Job drawing, mm, ordinate dimensions from the low corner. One solid piece. A direction names the side the tool comes from. Give positions to 0.01 mm unless a question says otherwise; leave off trailing zeros. Loops run counter-clockwise (first coordinate to the right, second up) from the corner with the lowest first, then second, coordinate; pieces in that order, holes last. Notation, with made-up numbers: M 71.25,15 L 98.25,15 A8 cw 98.25,27 Z; hole C -17.5,73 d9. An arc over 180 degrees is marked long. One line per question, with ' | ' between items.
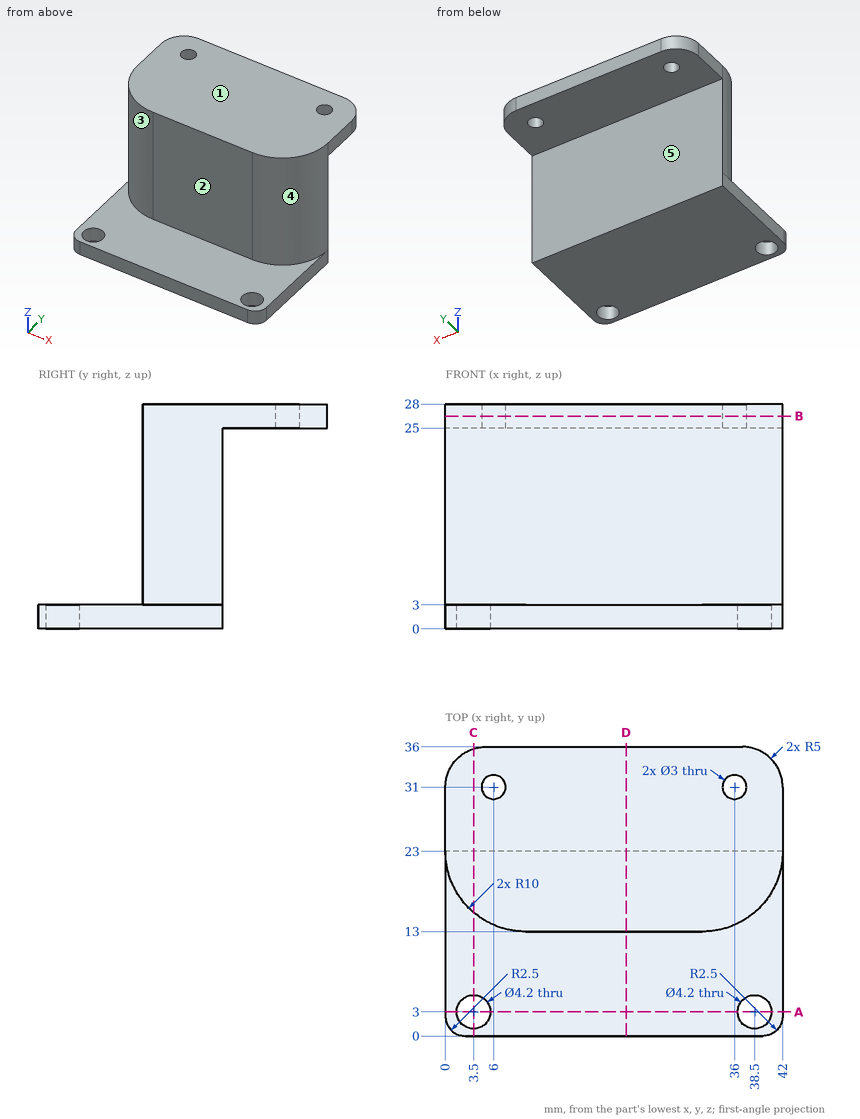
Item 1: Saw through at C-C on x = 3.5. Give the cut face in (y, z), and give its area (3 significant figures).
Conclusion:
outline: M 0,0 L 0.9,0 L 0.9,3 L 0,3 Z; M 5.1,0 L 23,0 L 23,25 L 35.77,25 L 35.77,28 L 15.4,28 L 15.4,3 L 5.1,3 Z | area: 285 mm²
Item 2: Saw through at B-B on z = 26.5. Give the cut face in (x, y), and give its area (3 significant figures).
Conclusion:
outline: M 0,23 A10 ccw 10,13 L 32,13 A10 ccw 42,23 L 42,31 A5 ccw 37,36 L 5,36 A5 ccw 0,31 Z; hole C 6,31 d3; hole C 36,31 d3 | area: 898 mm²
Item 3: Saw through at A-A on y = 3. Give the cut face in (x, z), and give its area (3 significant figures).
Conclusion:
outline: M 0,0 L 1.4,0 L 1.4,3 L 0,3 Z; M 5.6,0 L 36.4,0 L 36.4,3 L 5.6,3 Z; M 40.6,0 L 42,0 L 42,3 L 40.6,3 Z | area: 101 mm²
Item 4: 3-axis set-ups, long thin cutter, end or side, ignore diameter. For the marked faces 1, 2, 3, 4 and 5: which of +Z, -Z, +X, -X, +Y, -Y reach the whole face in a straight line?
Conclusion:
face 1: +Z, +X, -X, +Y, -Y | face 2: +Z, +X, -X, -Y | face 3: +Z, -X, -Y | face 4: +Z, +X, -Y | face 5: -Z, +X, -X, +Y
Item 5: Drill centre lines: line 1 along Y through (x, z) = (38.5, 0.95); line 2 along Z through (x, y) = (8, 33.5); line 3 along Z through (x, y) = (5, 5). Where is each one in solid material? Low to high. Write a range as [from, to].
Conclusion:
line 1: [0, 0.9], [5.1, 23] | line 2: [25, 28] | line 3: [0, 3]
Item 6: Drop flat-ended pins along their axis: P1, Ø4, axis at x = 31, y = 28.5, coming from the -Z side; P2, Ø12.5, axis at x = 13.5, z = 18, coming from the +Y side; P3, Ø1, axis at x = 26.5, y = 7, coming from the +Z side; P4, Ø1.8, axis at x = 6, y = 31, coming from the -Z side. Give the stop position or say it passes through.
Conclusion:
P1: z = 25 | P2: y = 23 | P3: z = 3 | P4: through
Item 7: Saw through at D-D on x = 22.5. Give the cut face in (y, z).
Conclusion:
outline: M 0,0 L 23,0 L 23,25 L 36,25 L 36,28 L 13,28 L 13,3 L 0,3 Z
